Part model, mm, in its own coordinate system. Round coordinates to 2 decimals unless told otherwise and drop trailing zeros. Write each loop counter-clockwise with the first axis right and the second up, starting at its lowest first coordinate (ties: lowest second). Pieces come first, ordered by that corner, then holes. Notation, with made-up numbers: M 82.5,56.5 L 110.5,56.5 A23 cw 110.5,89.5 Z; hole C 87,-19 d10. An arc over 180 degrees is marked long. Use a Markdown table: item, result. Add a question column.
1) Drop flat-ended pins along their axis: P1, Ø8.5, axis at x = 0, y = -36.5, coming from the +Z side; P2, Ø4, axis at x = -1, y = 29, coming from the -Z side; P3, Ø8, axis at x = -0.5, y = 6, coming from the +Z side. Give the stop position or say it passes through.
2) Slice it at B-B on y = 21. Write the cut outline in (x, z).
3) Wall check: probe 1 along X at (y, z) = (-36.5, 4.25); probe 2 along Z at (x, y) = (-2.75, -23.5); probe 3 along Y at (x, z) = (0, 5.75). Give the ranges that are in metal, low to high.
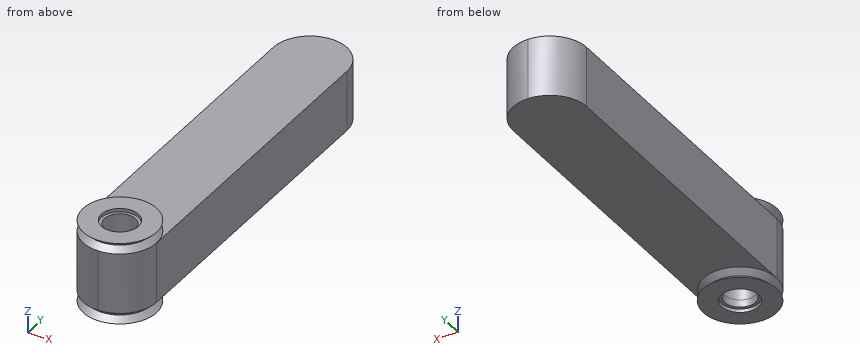
```python
from build123d import *

# Parameters (mm, degrees)
SKETCH_1_W          = 17
SKETCH_1_H          = 90
SKETCH_1_R          = 3.6
EXTRUDE_1_DEPTH     = 7
FILLET_1_R          = 8.5
SKETCH_2_R          = 8.5
SKETCH_2_R_2        = 3.6
EXTRUDE_2_DEPTH     = 2.5
SKETCH_4_R          = 4.3
CUT_EXTRUDE_1_DEPTH = 0.8


with BuildPart() as part:
    # 스케치1 → 보스-돌출1 (new, symmetric)
    with BuildSketch(Plane.XY):
        Rectangle(SKETCH_1_W, SKETCH_1_H)
        with Locations((0, -36.5)):
            Circle(SKETCH_1_R, mode=Mode.SUBTRACT)
    extrude(amount=EXTRUDE_1_DEPTH, both=True)

    # 필렛1
    fillet_1_edges = [part.edges().sort_by_distance(p)[0] for p in [
        (8.5, -45, 0),
        (-8.5, -45, 0),
        (-8.5, 45, 0),
        (8.5, 45, 0),
    ]]
    fillet(fillet_1_edges, radius=FILLET_1_R - 0.0001)  # a hair under: the kernel refuses the full size

    # 스케치2 → 보스-돌출2 (add)
    with BuildSketch(Plane.XY.offset(7)):
        with Locations((0, -36.5)):
            Circle(SKETCH_2_R)
        with Locations((0, -36.5)):
            Circle(SKETCH_2_R_2, mode=Mode.SUBTRACT)
    extrude_2 = extrude(amount=EXTRUDE_2_DEPTH)

    # 스케치3 → 컷-회전1 (revolve, cut)
    with BuildSketch(Plane(origin=(0, 0, 0), x_dir=(0, 0, -1), z_dir=(1, 0, 0)), mode=Mode.PRIVATE) as cut_revolve_1_sk:
        Polygon((-9.5, -28), (-8.25, -29.35), (-7, -28), align=None)
    cut_revolve_1 = revolve(cut_revolve_1_sk.sketch.rotate(Axis((0, -36.5, 0), (0, 0, 1)), 90), axis=Axis((0, -36.5, 0), (0, 0, 1)), mode=Mode.SUBTRACT)

    # 스케치4 → 컷-돌출1 (cut)
    with BuildSketch(Plane.XY.offset(9.5)):
        with Locations((0, -36.5)):
            Circle(SKETCH_4_R)
    cut_extrude_1 = extrude(amount=-CUT_EXTRUDE_1_DEPTH, mode=Mode.SUBTRACT)

    # 대칭 복사1: 보스-돌출2, 컷-회전1, 컷-돌출1 across plane
    add(extrude_2.mirror(Plane.XY))
    add(cut_revolve_1.mirror(Plane.XY), mode=Mode.SUBTRACT)
    add(cut_extrude_1.mirror(Plane.XY), mode=Mode.SUBTRACT)


solid = part.part
```
Entries:
| question | item | result |
|---|---|---|
| 1 | P1 | stops at z = 8.7 |
| 1 | P2 | stops at z = -7 |
| 1 | P3 | stops at z = 7 |
| 2 | outline | M -8.5,-7 L 8.5,-7 L 8.5,7 L -8.5,7 Z |
| 3 | probe 1 | x = -8.5 to -3.6, 3.6 to 8.5 |
| 3 | probe 2 | z = -7 to 7 |
| 3 | probe 3 | y = -45 to -40.1, -32.9 to 45 |
